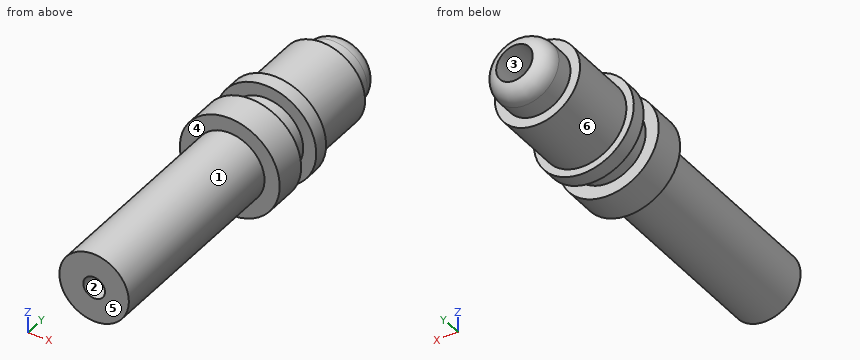
```python
from build123d import *

# Parameters (mm, degrees)
SKETCH1_R           = 5.75
BOSS_EXTRUDE1_DEPTH = 16
SKETCH2_OUTSIDE_W   = 18.062
SKETCH2_OUTSIDE_H   = 18.062
SKETCH2_OUTSIDE_R   = 4.9
CUT_EXTRUDE1_DEPTH  = 8
SKETCH3_R           = 3.8
BOSS_EXTRUDE2_DEPTH = 4
FILLET2_R           = 2
SKETCH4_R           = 4
BOSS_EXTRUDE3_DEPTH = 23.4
SKETCH12_W          = 1.5
SKETCH12_H          = 2.6
CUT_EXTRUDE2_REACH  = 46.155
SKETCH5_R           = 1.25
SKETCH13_R          = 2.1
CUT_EXTRUDE3_DEPTH  = 12


with BuildPart() as part:
    # Sketch1 → Boss-Extrude1 (new body)
    with BuildSketch(Plane(origin=(0, 0, 0), x_dir=(1, 0, 0), z_dir=(0, 1, 0))):
        with Locations(Location((0, 0, 0), (0, 0, 270))):
            Circle(SKETCH1_R)
    extrude(amount=BOSS_EXTRUDE1_DEPTH)

    # Sketch2 outside → Cut-Extrude1 (cut)
    with BuildSketch(Plane(origin=(0, 16, 0), x_dir=(1, 0, 0), z_dir=(0, 1, 0))):
        Rectangle(SKETCH2_OUTSIDE_W, SKETCH2_OUTSIDE_H)
        with Locations(Location((0, 0, 0), (0, 0, 270))):
            Circle(SKETCH2_OUTSIDE_R, mode=Mode.SUBTRACT)
    extrude(amount=-CUT_EXTRUDE1_DEPTH, mode=Mode.SUBTRACT)

    # Sketch3 → Boss-Extrude2 (add)
    with BuildSketch(Plane(origin=(0, 16, 0), x_dir=(1, 0, 0), z_dir=(0, 1, 0))):
        with Locations(Location((0, 0, 0), (0, 0, 270))):
            Circle(SKETCH3_R)
    extrude(amount=BOSS_EXTRUDE2_DEPTH)

    # Fillet2
    fillet2_edges = [part.edges().sort_by_distance(p)[0] for p in [
        (0, 20, -3.8),
    ]]
    fillet(fillet2_edges, radius=FILLET2_R)

    # Sketch4 → Boss-Extrude3 (add)
    with BuildSketch(Plane.XZ):
        with Locations(Location((0, 0, 0), (0, 0, 270))):
            Circle(SKETCH4_R)
    extrude(amount=BOSS_EXTRUDE3_DEPTH)

    # Sketch12 → Cut-Revolve2 (revolve, cut)
    with BuildSketch(Plane(origin=(0, 0, 0), x_dir=(0, 0, -1), z_dir=(1, 0, 0))):
        with Locations((-5, 5)):
            Rectangle(SKETCH12_W, SKETCH12_H)
    revolve(axis=Axis((0, 8, 0), (0, -1, 0)), mode=Mode.SUBTRACT)

    # Sketch5 → Cut-Extrude2 (cut, up to next)
    with BuildSketch(Plane.XZ.offset(23.4), mode=Mode.PRIVATE) as cut_extrude2_sk1:
        with Locations(Location((0, 0, 0), (0, 0, 270))):
            Circle(SKETCH5_R)
    cut_extrude2_tool1 = extrude(cut_extrude2_sk1.sketch, amount=-CUT_EXTRUDE2_REACH, mode=Mode.PRIVATE) & part.part
    add(cut_extrude2_tool1.solids().sort_by_distance((0, -23.4, 0))[0], mode=Mode.SUBTRACT)

    # Sketch13 → Cut-Extrude3 (cut)
    with BuildSketch(Plane(origin=(0, 20, 0), x_dir=(1, 0, 0), z_dir=(0, 1, 0))):
        with Locations(Location((0, 0, 0), (0, 0, 270))):
            Circle(SKETCH13_R)
    extrude(amount=-CUT_EXTRUDE3_DEPTH, mode=Mode.SUBTRACT)


solid = part.part
```
Model file for the job. Use its own axes, mm. Face numbers are marked on the shaded views. A direction names the side the tool comes from. Round coordinates to 2 decimals unless told otherwise and drop trailing zeros. Write each loop counter-clockwise with the first axis right and the second up, starting at its lowest first coordinate (ties: lowest second). Pieces come first, ordered by that corner, then holes. Notation, with made-up numbers: (86.25, 52.5) - (120.25, 52.5) arc R12 ccw to (120.25, 73.5) - close; hole circle Ø7 at (-6, 79). An arc over 180 degrees is marked (long way). One line per item, written item: value.
(1) Cut at A-A, the plane y = 1.5. Give the cut face in (x, z), plus the area to 3 significant figures.
Values follow:
outline: circle Ø11.5 at (0, 0); hole circle Ø2.5 at (0, 0)
area: 99.0 mm²
(2) Cut at B-B, the plane y = -17.5. Give the cut face in (x, z), plus the area to 3 significant figures.
Values follow:
outline: circle Ø8 at (0, 0); hole circle Ø2.5 at (0, 0)
area: 45.4 mm²
(3) Drop flat-ended pins along their axis: P1, Ø3, axis at x = 2.5, z = 0.5, coming from the +Y side; P2, Ø1, axis at x = -1.5, y = -6.5, coming from the +Z side; P3, Ø6, axis at y = -7.5, z = -2.5, coming from the -X side; P4, Ø2, axis at x = 0.5, z = 0, coming from the +Y side. Give the stop position or say it passes through.
Values follow:
P1: stops at y = 19.98
P2: stops at z = 3.87
P3: stops at x = -4
P4: stops at y = 8
(4) Two-plate mould, pull along X, no slides. Class the marked faces 1, 2, 3 and 4: pulls with the +X half, pulls with the -X half, needs draft (parallel to the pull), parting line crosses it, or undercut.
Values follow:
face 1: parting line crosses it
face 2: undercut
face 3: undercut
face 4: needs draft
(5) Wall check: probe 1 along Y at (x, z) = (-4.5, -3); probe 2 along X at (y, z) = (17.5, 0); probe 3 along X at (y, z) = (-2.5, 0). Give the ranges that are in metal, low to high.
Values follow:
probe 1: y = 0 to 3.7, 6.3 to 8
probe 2: x = -3.8 to -2.1, 2.1 to 3.8
probe 3: x = -4 to -1.25, 1.25 to 4
(6) 3-axis set-ups, long thin cutter, end or side, ignore diameter. For the marked faces 5 and 6: which of +Z, -Z, +X, -X, +Y, -Y reach the whole face in a straight line?
Values follow:
face 5: +Z, -Z, +X, -X, -Y
face 6: +Y
